from build123d import *

# Parameters (mm, degrees)
F0_W     = 4
F0_H     = 8
F1_DEPTH = 20


with BuildPart() as f1:
    # F0 (on Top) → F1 (new body)
    with BuildSketch(Plane.XY):
        Polygon((-20, -35), (0, -35), (0, 0), (2, 0), (2, -5), (4, -5), (4, 3), (-113, 3), (-117, 3), (-137, 3), (-141, 3), (-141, -27), (-138, -27), (-138, -7), align=None)
        with Locations((-139, 7)):
            Rectangle(F0_W, F0_H)
        with Locations((-115, 7)):
            Rectangle(F0_W, F0_H)
    extrude(amount=F1_DEPTH)


solid = f1.part
Could you check a few things on this model? Use its own coordinates, in mm. A direction names the side the tool comes from. Give positions to 0.01 mm unless a question says otherwise; leave off trailing zeros. Loops run counter-clockwise (first coordinate to the right, second up) from the corner with the lowest first, then second, coordinate; pieces in that order, holes last. Notation, with made-up numbers: (-28.5, 5.25) -> (-7.5, 5.25) arc R33 cw to (-7.5, 33.25) -> close; hole circle Ø6 at (84, -8). An arc over 180 degrees is marked (long way). Answer as CSV lines item,"result". Start each with the question number.
(1) We'd pull the mould along X, two halves only. Please class faces 6 (the flat face through (4, -1, 10)), 7 (the flat face through (-141, -8, 10)), 8 (the flat face through (-140, -27, 10)), 9 (the flat face through (-79.826, -20.804, 9.86)): released by +X, released by -X, zero draft, split by the parting line, or undercut.
(2) If we section it at B-B on z = 12.75: Write out the boundary of the cut face in (x, y), then the cut area to 3 significant figures.
(3) I need wall thicknesses on probe 1 along X at (y, z) = (6, 7.75); probe 2 along X at (y, z) = (-2.5, 16.5); probe 3 along Y at (x, z) = (-117.5, 8.75). Which ranges of each line are inside material? Lowest first, please.
(4) If we section it at D-D on y = -30.5: Write out the boundary of the cut face in (x, z), then the cut area to 3 significant figures.
(5) I'm going to push flat-ended pins straight in: pin 1 Ø0.6 at (x, z) = (3, 10) entering from -Y; pin 2 Ø2.5 at (y, z) = (7.5, 5.5) entering from +X; pin 3 Ø8 at (x, z) = (-78, 8.5) entering from +Y. Where does each tip first touch, or does it pass through?
(6) Which directions (+Z, -Z, +X, -X, +Y, -Y) give clear straight access to the entire face, cutting with the end or side of a thin tool? Please do faces 1 (the flat face through (-139, 11, 10)), 2 (the flat face through (-53, -12, 0)), 3 (the flat face through (-54, 3, 10)), 4 (the flat face through (-127, 3, 10)), 5 (the flat face through (2, -2, 10)).
(7) If we section it at C-C on x = -11.5: Write out the boundary of the cut face in (y, z), then the cut area to 3 significant figures.
(8) If we section it at A-A on y = -11.5: Write out the boundary of the cut face in (x, z).
Computed:
1,face 6,"released by +X"
1,face 7,"released by -X"
1,face 8,"zero draft"
1,face 9,"undercut"
2,outline,"(-141, -27) -> (-138, -27) -> (-138, -7) -> (-20, -35) -> (0, -35) -> (0, 0) -> (2, 0) -> (2, -5) -> (4, -5) -> (4, 3) -> (-113, 3) -> (-113, 11) -> (-117, 11) -> (-117, 3) -> (-137, 3) -> (-137, 11) -> (-141, 11) -> close"
2,area,"3,770 mm2"
3,probe 1,"x = -141 to -137, -117 to -113"
3,probe 2,"x = -141 to 0, 2 to 4"
3,probe 3,"y = -11.86 to 3"
4,outline,"(-38.96, 0) -> (0, 0) -> (0, 20) -> (-38.96, 20) -> close"
4,area,"779 mm2"
5,pin 1,"stops at y = -5"
5,pin 2,"stops at x = -113"
5,pin 3,"stops at y = 3"
6,face 1,"+Z, -Z, +X, -X, +Y"
6,face 2,"-Z, +X, -X, +Y, -Y"
6,face 3,"+Z, -Z, +X, +Y"
6,face 4,"+Z, -Z, +Y"
6,face 5,"+Z, -Z, -Y"
7,outline,"(-35, 0) -> (3, 0) -> (3, 20) -> (-35, 20) -> close"
7,area,"760 mm2"
8,outline,"(-141, 0) -> (-138, 0) -> (-138, 20) -> (-141, 20) -> close; (-119.04, 0) -> (0, 0) -> (0, 20) -> (-119.04, 20) -> close"
